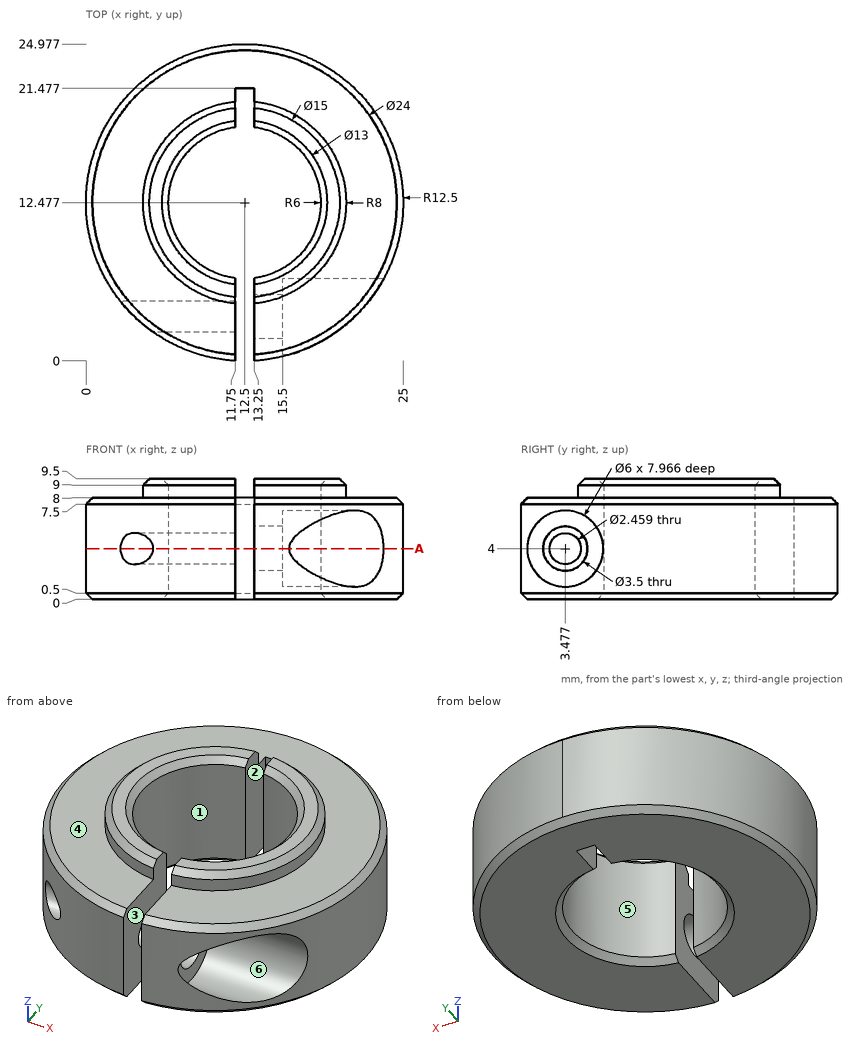
Geometry check sheet. Reference: drawing and pictorial views, mm from the part's lowest x, y, z. A direction names the side the tool comes from. Round coordinates to 2 decimals unless told otherwise and drop trailing zeros. Use a Markdown table: item, result. Add a question column.
1) Gauge pin test, flat ends, axial feed: P1, Ø3, axis at x = 11, y = 9.5, coming from the -Z side; P2, Ø5, axis at y = 2.5, z = 3.5, coming from the -X side; P3, Ø5, axis at y = 3.48, z = 4, coming from the +X side; P4, Ø1, axis at x = 8, z = 3, coming from the -Y side (1 decimal). Record the tip position at first contact, or that the pin passes through.
2) Section check A-A (z = 4). Count the separate pieces of the cut face and the enclosed holes in it, then the cut area to 3 significant figures.
3) Set-up check for the marked faces 3, 4, 5 and 6: record each of +Z, -Z, +X, -X, +Y, -Y from which the full face is reachable in a straight line by a thin tool's end or side.
4) Thickness scan on line 1 along Y through (x, z) = (16.25, 6) (1 decimal); line 2 along Z through (x, y) = (3.5, 18); line 3 along X through (y, z) = (13.5, 1). Record the ranges inside material, lowest first.
5) Mould release check, pull along Y, two halves, no side actions. Record for the marked faces 1 and 2: released by +Y, released by -Y, zero draft, split by the parting line, or undercut.
Established:
| question | item | result |
|---|---|---|
| 1 | P1 | through |
| 1 | P2 | x = 2.48 |
| 1 | P3 | x = 15.5 |
| 1 | P4 | y = 0.6 |
| 2 | separate pieces | 3 |
| 2 | enclosed holes | 0 |
| 2 | area | 305 mm2 |
| 3 | face 3 | +Z, -Z, -Y |
| 3 | face 4 | +Z |
| 3 | face 5 | +Z, -Z |
| 3 | face 6 | +X |
| 4 | line 1 | 0.6 to 1.2, 5.7 to 7.8, 17.2 to 24.4 |
| 4 | line 2 | 0 to 8 |
| 4 | line 3 | 0.04 to 6.59, 18.41 to 24.96 |
| 5 | face 1 | undercut |
| 5 | face 2 | zero draft |
